from build123d import *

# Parameters (mm, degrees)
F1_DEPTH = 62
F2_DEPTH = 12
F4_D     = 12
F4_DEPTH = 8
F4_TIP   = 3.6051637142
F6_D     = 16
F6_DEPTH = 8
F6_TIP   = 4.8068849522
F7_D     = 4
F7_DEPTH = 8
F7_TIP   = 1.2017212381
F8_D     = 14
F8_DEPTH = 8
F8_TIP   = 4.2060243332


with BuildPart() as f1:
    # F0 (on Top) → F1 (new body)
    with BuildSketch(Plane.XY):
        with BuildLine():
            ThreePointArc((65, 60), (63.5355339059, 63.5355339059), (60, 65))
            Line((60, 65), (-60, 65))
            ThreePointArc((-60, 65), (-63.5355339059, 63.5355339059), (-65, 60))
            Line((-65, 60), (-65, -60))
            ThreePointArc((-65, -60), (-63.5355339059, -63.5355339059), (-60, -65))
            Line((-60, -65), (60, -65))
            ThreePointArc((60, -65), (63.5355339059, -63.5355339059), (65, -60))
            Line((65, -60), (65, 60))
        make_face()
        with BuildLine():
            Line((-57, 62), (57, 62))
            ThreePointArc((57, 62), (60.5355339059, 60.5355339059), (62, 57))
            Line((62, 57), (62, -57))
            ThreePointArc((62, -57), (60.5355339059, -60.5355339059), (57, -62))
            Line((57, -62), (-57, -62))
            ThreePointArc((-57, -62), (-60.5355339059, -60.5355339059), (-62, -57))
            Line((-62, -57), (-62, 57))
            ThreePointArc((-62, 57), (-60.5355339059, 60.5355339059), (-57, 62))
        make_face(mode=Mode.SUBTRACT)
    extrude(amount=F1_DEPTH)

    # F0 (on Top) → F2 (join)
    with BuildSketch(Plane.XY):
        with BuildLine():
            ThreePointArc((62, 57), (60.5355339059, 60.5355339059), (57, 62))
            Line((57, 62), (-57, 62))
            ThreePointArc((-57, 62), (-60.5355339059, 60.5355339059), (-62, 57))
            Line((-62, 57), (-62, -57))
            ThreePointArc((-62, -57), (-60.5355339059, -60.5355339059), (-57, -62))
            Line((-57, -62), (57, -62))
            ThreePointArc((57, -62), (60.5355339059, -60.5355339059), (62, -57))
            Line((62, -57), (62, 57))
        make_face()
    extrude(amount=F2_DEPTH)

    # F4
    with Locations(Plane(origin=(0, 65, 0), x_dir=(-1, 0, 0), z_dir=(0, 1, 0))):
        with Locations((-32.5, 29.5), (0, 29.5), (32.5, 29.5)):
            Hole(F4_D / 2, depth=F4_DEPTH)
            with Locations((0, 0, -(F4_DEPTH + F4_TIP / 2))):  # 118° drill point
                Cone(0, F4_D / 2, F4_TIP, mode=Mode.SUBTRACT)

    # F6
    with Locations(Plane.XZ.offset(65)):
        with Locations((-32.5, 29.5)):
            Hole(F6_D / 2, depth=F6_DEPTH)
            with Locations((0, 0, -(F6_DEPTH + F6_TIP / 2))):  # 118° drill point
                Cone(0, F6_D / 2, F6_TIP, mode=Mode.SUBTRACT)

    # F7
    with Locations(Plane.XZ.offset(65)):
        with Locations((0, 13)):
            Hole(F7_D / 2, depth=F7_DEPTH)
            with Locations((0, 0, -(F7_DEPTH + F7_TIP / 2))):  # 118° drill point
                Cone(0, F7_D / 2, F7_TIP, mode=Mode.SUBTRACT)

    # F8
    with Locations(Plane.XZ.offset(65)):
        with Locations((32.5, 29.5)):
            Hole(F8_D / 2, depth=F8_DEPTH)
            with Locations((0, 0, -(F8_DEPTH + F8_TIP / 2))):  # 118° drill point
                Cone(0, F8_D / 2, F8_TIP, mode=Mode.SUBTRACT)


solid = f1.part
Can you work these out from the model? Positions are in its coordinate system, mm. A direction names the side the tool comes from. Coordinates: 2 decimals unless noted, no trailing zeros. Loops run counter-clockwise (first coordinate to the right, second up) from the corner with the lowest first, then second, coordinate; pieces in that order, holes last. Notation, with made-up numbers: M 35.25,51 L 63.25,51 A22 ccw 63.25,65 Z; hole C 39.5,76.5 d5. An arc over 180 degrees is marked long. Answer as CSV lines item,"result". Start each with the question number.
1. Thinking about a two-plate mould opening in X: for faces 1 (the face through (-62, -1, 37)), 2 (the face through (1, 65, 37)), 3 (the face through (-63, 64, 31)), which applies, +X half, -X half, draft (parallel to the pull), parting line (faces both ways), or undercut?
2. For pin 1 Ø5 at (x, y) = (16, 33) entering from -Z; pin 2 Ø7 at (x, z) = (-32.5, 29.5) entering from +Y, each with a flat end and sliding along its axis, tell me the tip position at first contact or that it passes through.
3. Suppose I cut it at B-B, the plane z = 48. List the corners of the cut face in (x, y) for me, plus the area to 3 significant figures.
4. Suppose I cut it at C-C, the plane x = -16. List the corners of the cut face in (y, z) for me.
5. For faces 4 (the face through (-1.301, 63.479, 23.643)), 5 (the face through (-1, -65, 31)), 6 (the face through (-26.6, -63.5, 34.9)), 7 (the face through (-1, 62, 37)), which set-ups out of +Z, -Z, +X, -X, +Y, -Y let a thin tool reach every point of the face, with its end or its side?
6. If I drill on probe 1 along Z at (x, y) = (0, -62.25); probe 2 along Y at (x, z) = (41, 32), over which ranges is the centre line in solid material (lowest first)? Write a range as [from, to].
7. Suppose I cut it at A-A, the plane x = -32.5. List the corners of the cut face in (y, z) for me, plus the area to 3 significant figures.
Output:
1,face 1,"undercut"
1,face 2,"draft"
1,face 3,"-X half"
2,pin 1,"stops at z = 0"
2,pin 2,"passes through"
3,outline,"M -65,-60 A5 ccw -60,-65 L 60,-65 A5 ccw 65,-60 L 65,60 A5 ccw 60,65 L -60,65 A5 ccw -65,60 Z; hole M -62,-57 A5 ccw -57,-62 L 57,-62 A5 ccw 62,-57 L 62,57 A5 ccw 57,62 L -57,62 A5 ccw -62,57 Z"
3,area,"1,520 mm^2"
4,outline,"M -65,0 L 65,0 L 65,62 L 62,62 L 62,12 L -62,12 L -62,62 L -65,62 Z"
5,face 4,"+Y"
5,face 5,"+Z, -Z, +X, -X, -Y"
5,face 6,"-Y"
5,face 7,"+Z"
6,probe 1,"z = [0, 11], [15, 62]"
6,probe 2,"y = [-65, -62], [62, 65]"
7,outline,"M -65,0 L 65,0 L 65,23.5 L 62,23.5 L 62,12 L -62,12 L -62,21.5 L -65,21.5 Z; M -65,37.5 L -62,37.5 L -62,62 L -65,62 Z; M 62,35.5 L 65,35.5 L 65,62 L 62,62 Z"
7,area,"1,780 mm^2"
